Can you work these out from the drawing? Everything is in mm from the part's minimum corner. A direction names the side the tool comes from. Round coordinates to 2 decimals unless told otherwise and drop trailing zeros. Loops run counter-clockwise (first coordinate to the right, second up) from the corner with the lowest first, then second, coordinate; pieces in that order, holes last. Notation, with made-up numbers: M -25.5,42 L -5.5,42 A19 ccw -5.5,50 Z; hole C -13,66.5 d11. An arc over 180 degrees is marked long. Answer in a Markdown table with one row per item.
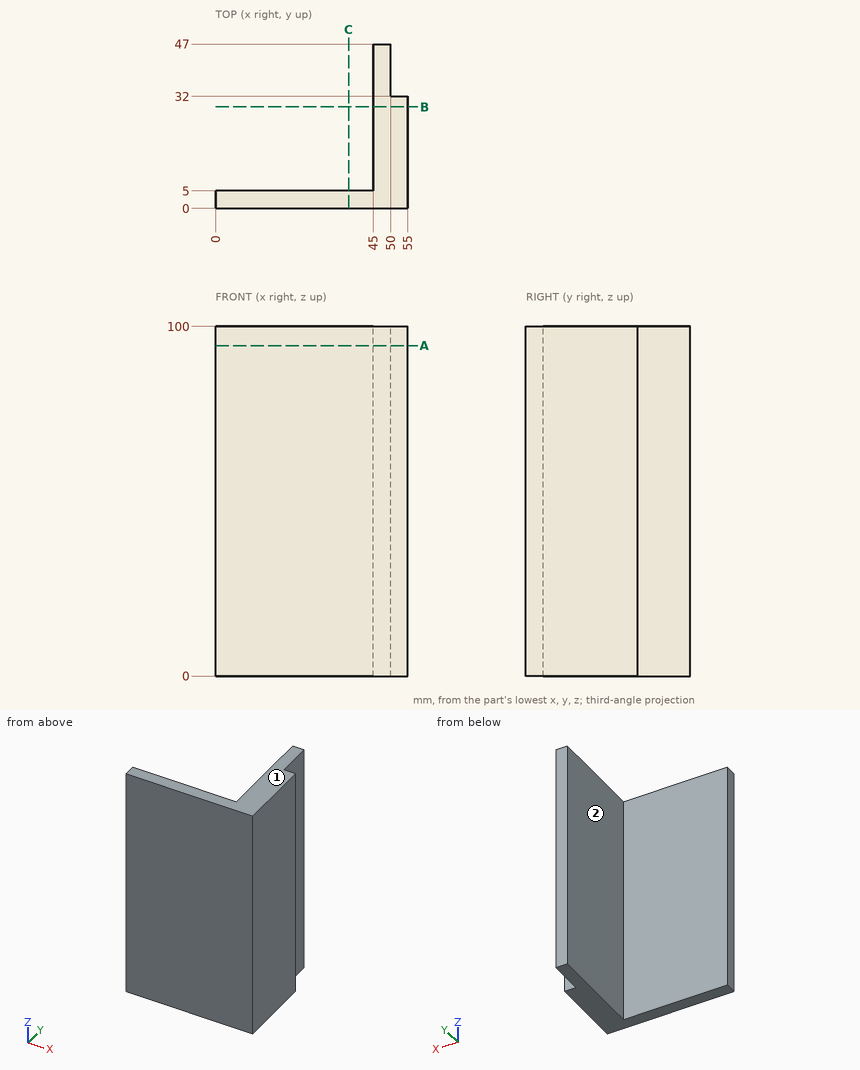
1) I want a section at C-C, the plane x = 38. Please give me the cut outline in (y, z).
Computed:
| item | result |
|---|---|
| outline | M 0,0 L 5,0 L 5,100 L 0,100 Z |
2) I need wall thicknesses on line 1 (X direction, y = 10, z = 43); line 2 (Y direction, x = 23, z = 49); line 3 (X direction, y = 43, z = 49). Which ranges of each line are inside material? Lowest first, please.
Computed:
| item | result |
|---|---|
| line 1 | x = 45 to 55 |
| line 2 | y = 0 to 5 |
| line 3 | x = 45 to 50 |
3) I want a section at A-A, the plane z = 94.5. Please give me the cut outline in (x, y), plus the area to 3 significant figures.
Computed:
| item | result |
|---|---|
| outline | M 0,0 L 55,0 L 55,32 L 50,32 L 50,47 L 45,47 L 45,5 L 0,5 Z |
| area | 620 mm² |
4) Which directions (+Z, -Z, +X, -X, +Y, -Y) give clear straight access to the entire face, cutting with the end or side of a thin tool? Please do the marked faces 1 and 2.
Computed:
| item | result |
|---|---|
| face 1 | +Z, +X, -X, +Y, -Y |
| face 2 | +Z, -Z, -X, +Y |
5) I want a section at B-B, the plane y = 29. Please give me the cut outline in (x, z), plus the area to 3 significant figures.
Computed:
| item | result |
|---|---|
| outline | M 45,0 L 55,0 L 55,100 L 45,100 Z |
| area | 1,000 mm² |
6) Will these pins go through, and if not, where does the flat tip stop? P1, Ø12, axis at y = 42, z = 27, coming from the +X side; P2, Ø8, axis at y = 15.5, z = 79, coming from the -X side; P3, Ø12, axis at x = 35, y = 25, coming from the -Z side; P4, Ø4, axis at x = 24.5, z = 87, coming from the +Y side.
Computed:
| item | result |
|---|---|
| P1 | stops at x = 50 |
| P2 | stops at x = 45 |
| P3 | passes through |
| P4 | stops at y = 5 |
